Check sheet for the modelled part. Datum: model origin and axes. Units: mm. A direction names the side the tool comes from. Give positions to 0.01 mm unless a question says otherwise; leave off trailing zeros. Loops run counter-clockwise (first coordinate to the right, second up) from the corner with the lowest first, then second, coordinate; pieces in that order, holes last.
Autodesk Inventor part; units mm, degrees
ref_plane "YZ Plane" through (0, 0, 0) normal (1, 0, 0) x (0, 1, 0)
ref_plane "XZ Plane" through (0, 0, 0) normal (0, 1, 0) x (-1, 0, 0)
ref_plane "XY Plane" through (0, 0, 0) normal (0, 0, 1) x (1, 0, 0)
sketch "草圖1" plane through (0, 0, 0) normal (0, 0, 1) x (1, 0, 0)
  circle A0 centre (0, 0) radius 30
  dimension "d0" = 60
extrude "擠出1" add sketch "草圖1" along normal blind 5
sketch "草圖2" plane through (0, 0, 5) normal (0, 0, 1) x (1, 0, 0)
  circle A0 centre (0, 20) radius 3
  circle A1 centre (-17.3205, 10) radius 3
  circle A2 centre (-17.3205, -10) radius 3
  circle A3 centre (0, -20) radius 3
  circle A4 centre (17.3205, -10) radius 3
  circle A5 centre (17.3205, 10) radius 3
  point P0 (0, 0)
  dimension "d4" = 6
  dimension "d5" = 20
  dimension "d8" = 360
extrude "擠出2" add sketch "草圖2" along normal blind 5
sketch "草圖3" plane through (0, 0, 0) normal (0, 0, -1) x (-1, 0, 0)
  circle A0 centre (0, 0) radius 5
  dimension "d12" = 10
extrude "擠出3" add sketch "草圖3" along normal blind 20
properties part number "Output_Shaft"
(1) Section check D-D on z = -1.75. Record the boundary of the cut face in (x, y).
(2) Section check A-A on z = 7. Record the boundary of the cut face in (x, y).
(3) Section check B-B on y = 0. Record the boundary of the cut face in (x, z).
(4) Section check C-C on x = 0. Record the boundary of the cut face in (y, z).
(5) Gauge pin test, flat ends, axial feed: pin 1 Ø10 at (x, y) = (10.5, 10) entering from -Z; pin 2 Ø12 at (x, z) = (22, 5) entering from -Y; pin 3 Ø5 at (y, z) = (-13.5, 0) entering from -X; pin 4 Ø5 at (y, z) = (20, -3) entering from +X (3 decimals). Record the tip position at first contact, or that the pin passes through.
(6) Release check for a two-part mould opening along Y. For faces 3 (the face through (18.93, 7.47, 7.46)), 4 (the face through (1.08, 4.88, -9.86)), 5 (the face through (0, -6, 0)) record: pulls with the +Y half, pulls with the -Y half, needs draft (parallel to the pull), parting line crosses it, or undercut.
(7) Access from +Z, -Z, +X, -X, +Y, -Y to the whole of each face (thin tool, end or side, straight path). Record for faces 1 (the face through (-29.97, -1.32, 2.46)), 2 (the face through (-0.65, 22.93, 7.46)).
(8) Material ranges on line 1 (Z direction, x = -3.5, y = 3); line 2 (Z direction, x = 2.5, y = -24.5); line 3 (Y direction, x = -23, z = 1.5), recorded low to high.
Computed values:
1. outline: circle Ø10 at (0, 0)
2. outline: circle Ø6 at (-17.32, -10); circle Ø6 at (-17.32, 10); circle Ø6 at (0, -20); circle Ø6 at (0, 20); circle Ø6 at (17.32, -10); circle Ø6 at (17.32, 10)
3. outline: (-30, 0) - (-5, 0) - (-5, -20) - (5, -20) - (5, 0) - (30, 0) - (30, 5) - (-30, 5) - close
4. outline: (-30, 0) - (-5, 0) - (-5, -20) - (5, -20) - (5, 0) - (30, 0) - (30, 5) - (23, 5) - (23, 10) - (17, 10) - (17, 5) - (-17, 5) - (-17, 10) - (-23, 10) - (-23, 5) - (-30, 5) - close
5. pin 1: stops at z = 0
5. pin 2: stops at y = -25.38
5. pin 3: stops at x = -27.91
5. pin 4: passes through
6. face 3: undercut
6. face 4: parting line crosses it
6. face 5: needs draft
7. face 1: +Z, -Z
7. face 2: +Z
8. line 1: z = -20 to 5
8. line 2: z = 0 to 5
8. line 3: y = -19.26 to 19.26
